```python
from build123d import *

# Parameters (mm, degrees)
F0_W     = 102.87
F0_H     = 13.97
F0_W_2   = 12.3800332606
F0_H_2   = 12.7
F0_W_3   = 3.175
F0_H_3   = 5.08
F0_W_4   = 12.0600665212
F0_W_5   = 0.6399334788
F1_DEPTH = 2.54
F2_DEPTH = 6.35
F3_DEPTH = 3.175
F5_D     = 0.254
F5_DEPTH = 0.636
F6_D     = 0.254


with BuildPart() as f1:
    # F0 (on Top) → F1 (new body)
    with BuildSketch(Plane.XY):
        with Locations((18.0648645937, 6.35)):
            Rectangle(F0_W, F0_H)
        Polygon((-20.3551021457, 0), (-32.7351354063, 0), (-32.7351354063, 12.7), (-20.3551021457, 12.7), (-19.7151686668, 12.7), (-7.6551021457, 12.7), (-7.0151686668, 12.7), (5.0448978543, 12.7), (5.6848313332, 12.7), (17.7448978543, 12.7), (18.3848313332, 12.7), (30.4448978543, 12.7), (31.0848313332, 12.7), (43.1448978543, 12.7), (43.7848313332, 12.7), (55.8448978543, 12.7), (56.4848313332, 12.7), (68.8648645937, 12.7), (68.8648645937, 0), (56.4848313332, 0), (55.8448978543, 0), (43.7848313332, 0), (43.1448978543, 0), (31.0848313332, 0), (30.4448978543, 0), (18.3848313332, 0), (17.7448978543, 0), (5.6848313332, 0), (5.0448978543, 0), (-7.0151686668, 0), (-7.6551021457, 0), (-19.7151686668, 0), align=None, mode=Mode.SUBTRACT)
        with Locations((62.6748479635, 6.35)):
            Rectangle(F0_W_2, F0_H_2)
        with Locations((62.5148645937, 6.35)):
            Rectangle(F0_W_3, F0_H_3, mode=Mode.SUBTRACT)
        with Locations((-26.545118776, 6.35)):
            Rectangle(F0_W_2, F0_H_2)
        with Locations((-26.3851354063, 6.35)):
            Rectangle(F0_W_3, F0_H_3, mode=Mode.SUBTRACT)
        with Locations((-13.6851354063, 6.35)):
            Rectangle(F0_W_4, F0_H_2)
        with Locations((-13.6851354063, 6.35)):
            Rectangle(F0_W_3, F0_H_3, mode=Mode.SUBTRACT)
        with Locations((-0.9851354063, 6.35)):
            Rectangle(F0_W_4, F0_H_2)
        with Locations((-0.9851354063, 6.35)):
            Rectangle(F0_W_3, F0_H_3, mode=Mode.SUBTRACT)
        with Locations((49.8148645937, 6.35)):
            Rectangle(F0_W_4, F0_H_2)
        with Locations((49.8148645937, 6.35)):
            Rectangle(F0_W_3, F0_H_3, mode=Mode.SUBTRACT)
        with Locations((37.1148645937, 6.35)):
            Rectangle(F0_W_4, F0_H_2)
        with Locations((37.1148645937, 6.35)):
            Rectangle(F0_W_3, F0_H_3, mode=Mode.SUBTRACT)
        with Locations((11.7148645937, 6.35)):
            Rectangle(F0_W_4, F0_H_2)
        with Locations((11.7148645937, 6.35)):
            Rectangle(F0_W_3, F0_H_3, mode=Mode.SUBTRACT)
        with Locations((24.4148645937, 6.35)):
            Rectangle(F0_W_4, F0_H_2)
        with Locations((24.4148645937, 6.35)):
            Rectangle(F0_W_3, F0_H_3, mode=Mode.SUBTRACT)
        with Locations((49.8148645937, 6.35)):
            Rectangle(F0_W_3, F0_H_3)
        with Locations((24.4148645937, 6.35)):
            Rectangle(F0_W_3, F0_H_3)
        with Locations((-26.3851354063, 6.35)):
            Rectangle(F0_W_3, F0_H_3)
        with Locations((-0.9851354063, 6.35)):
            Rectangle(F0_W_3, F0_H_3)
        with Locations((-13.6851354063, 6.35)):
            Rectangle(F0_W_3, F0_H_3)
        with Locations((62.5148645937, 6.35)):
            Rectangle(F0_W_3, F0_H_3)
        with Locations((11.7148645937, 6.35)):
            Rectangle(F0_W_3, F0_H_3)
        with Locations((37.1148645937, 6.35)):
            Rectangle(F0_W_3, F0_H_3)
        with Locations((5.3648645937, 6.35)):
            Rectangle(F0_W_5, F0_H_2)
        with Locations((56.1648645937, 6.35)):
            Rectangle(F0_W_5, F0_H_2)
        with Locations((18.0648645937, 6.35)):
            Rectangle(F0_W_5, F0_H_2)
        with Locations((30.7648645937, 6.35)):
            Rectangle(F0_W_5, F0_H_2)
        with Locations((43.4648645937, 6.35)):
            Rectangle(F0_W_5, F0_H_2)
        with Locations((-7.3351354063, 6.35)):
            Rectangle(F0_W_5, F0_H_2)
        with Locations((-20.0351354063, 6.35)):
            Rectangle(F0_W_5, F0_H_2)
    extrude(amount=-F1_DEPTH)

    # F0 (on Top) → F2 (join)
    with BuildSketch(Plane.XY):
        with Locations((18.0648645937, 6.35)):
            Rectangle(F0_W, F0_H)
        Polygon((-20.3551021457, 0), (-32.7351354063, 0), (-32.7351354063, 12.7), (-20.3551021457, 12.7), (-19.7151686668, 12.7), (-7.6551021457, 12.7), (-7.0151686668, 12.7), (5.0448978543, 12.7), (5.6848313332, 12.7), (17.7448978543, 12.7), (18.3848313332, 12.7), (30.4448978543, 12.7), (31.0848313332, 12.7), (43.1448978543, 12.7), (43.7848313332, 12.7), (55.8448978543, 12.7), (56.4848313332, 12.7), (68.8648645937, 12.7), (68.8648645937, 0), (56.4848313332, 0), (55.8448978543, 0), (43.7848313332, 0), (43.1448978543, 0), (31.0848313332, 0), (30.4448978543, 0), (18.3848313332, 0), (17.7448978543, 0), (5.6848313332, 0), (5.0448978543, 0), (-7.0151686668, 0), (-7.6551021457, 0), (-19.7151686668, 0), align=None, mode=Mode.SUBTRACT)
    extrude(amount=F2_DEPTH)

    # F0 (on Top) → F3 (join)
    with BuildSketch(Plane.XY):
        with Locations((-26.3851354063, 6.35)):
            Rectangle(F0_W_3, F0_H_3)
        with Locations((-13.6851354063, 6.35)):
            Rectangle(F0_W_3, F0_H_3)
        with Locations((-0.9851354063, 6.35)):
            Rectangle(F0_W_3, F0_H_3)
        with Locations((11.7148645937, 6.35)):
            Rectangle(F0_W_3, F0_H_3)
        with Locations((24.4148645937, 6.35)):
            Rectangle(F0_W_3, F0_H_3)
        with Locations((37.1148645937, 6.35)):
            Rectangle(F0_W_3, F0_H_3)
        with Locations((49.8148645937, 6.35)):
            Rectangle(F0_W_3, F0_H_3)
        with Locations((62.5148645937, 6.35)):
            Rectangle(F0_W_3, F0_H_3)
        with Locations((56.1648645937, 6.35)):
            Rectangle(F0_W_5, F0_H_2)
        with Locations((43.4648645937, 6.35)):
            Rectangle(F0_W_5, F0_H_2)
        with Locations((30.7648645937, 6.35)):
            Rectangle(F0_W_5, F0_H_2)
        with Locations((18.0648645937, 6.35)):
            Rectangle(F0_W_5, F0_H_2)
        with Locations((5.3648645937, 6.35)):
            Rectangle(F0_W_5, F0_H_2)
        with Locations((-7.3351354063, 6.35)):
            Rectangle(F0_W_5, F0_H_2)
        with Locations((-20.0351354063, 6.35)):
            Rectangle(F0_W_5, F0_H_2)
    extrude(amount=F3_DEPTH)

    # F5 (through all, one way)
    with BuildSketch(Plane(origin=(0, 0, 0), x_dir=(-1, 0, 0), z_dir=(0, 1, 0))):
        with Locations((26.6391354063, 1.5875), (26.1311354063, 1.5875), (13.9391354063, 1.5875), (13.4311354063, 1.5875), (1.2391354063, 1.5875), (0.7311354063, 1.5875), (-11.4608645937, 1.5875), (-11.9688645937, 1.5875), (-24.1608645937, 1.5875), (-24.6688645937, 1.5875), (-36.8608645937, 1.5875), (-37.3688645937, 1.5875), (-49.5608645937, 1.5875), (-50.0688645937, 1.5875), (-62.2608645937, 1.5875), (-62.7688645937, 1.5875)):
            Circle(F5_D / 2)
    extrude(amount=-F5_DEPTH, mode=Mode.SUBTRACT)

    # F6 (through all)
    with Locations(Plane(origin=(0, 0, 0), x_dir=(-1, 0, 0), z_dir=(0, -1, 0))):
        with Locations((-62.7688645937, -1.5875), (-62.2608645937, -1.5875), (-50.0688645937, -1.5875), (-49.5608645937, -1.5875), (-37.3688645937, -1.5875), (-36.8608645937, -1.5875), (-24.6688645937, -1.5875), (-24.1608645937, -1.5875), (-11.9688645937, -1.5875), (-11.4608645937, -1.5875), (0.7311354063, -1.5875), (1.2391354063, -1.5875), (13.4311354063, -1.5875), (13.9391354063, -1.5875), (26.1311354063, -1.5875), (26.6391354063, -1.5875)):
            Hole(F6_D / 2)


solid = f1.part
```
The model under review builds one solid part; all positions refer to its coordinate system, in mm. A direction names the side the tool comes from. Give positions to 0.01 mm unless a question says otherwise; leave off trailing zeros. Write each loop counter-clockwise with the first axis right and the second up, starting at its lowest first coordinate (ties: lowest second). Pieces come first, ordered by that corner, then holes. Notation, with made-up numbers: (48.5, 89) -> (103.5, 89) arc R7 ccw to (103.5, 100) -> close; hole circle Ø3 at (77, 4.25). An arc over 180 degrees is marked (long way). Put each result on its own line as item: value.
(1) To check wall thickness, follow probe 1 along Y at (x, z) = (23, 0.25) (3 decimals); probe 2 along Y at (x, z) = (38.5, 4.75) (3 decimals); probe 3 along X at (y, z) = (10, 5). State the ranges of each line that lie inside material, in increasing order. Write a range as from..to.
Results are:
probe 1: -0.635..0, 3.81..8.89, 12.7..13.335
probe 2: -0.635..0, 12.7..13.335
probe 3: -33.37..-32.74, 68.86..69.5
(2) We need section B-B, the plane x = 53.5. Give the boundary of the cut face in (y, z) (3 decimals), and give its area (3 significant figures).
Results are:
outline: (-0.635, -2.54) -> (13.335, -2.54) -> (13.335, 6.35) -> (12.7, 6.35) -> (12.7, 0) -> (0, 0) -> (0, 6.35) -> (-0.635, 6.35) -> close
area: 43.5 mm²
(3) We need section C-C, the plane y = 7.25. State how many separate pieces and enclosed holes the cut face has, and give its area (3 significant figures).
Results are:
separate pieces: 1
enclosed holes: 16
area: 363 mm²
(4) We need section A-A, the plane z = 5.25. Give the boundary of the cut face in (x, y) (3 decimals).
Results are:
outline: (-33.37, -0.635) -> (69.5, -0.635) -> (69.5, 13.335) -> (-33.37, 13.335) -> close; hole (-32.735, 0) -> (68.865, 0) -> (68.865, 12.7) -> (-32.735, 12.7) -> close
(5) The part is to be moulded in two halves that separate along X. For faces 1 (the flat face through (17, -0.635, 2)), 2 (the flat face through (48.227, 6, 2)), say which applies: pulls with the +X half, pulls with the -X half, needs draft (parallel to the pull), parting line crosses it, or undercut.
Results are:
face 1: needs draft
face 2: undercut
(6) For pin 1 Ø1 at (x, y) = (-27, 6) entering from +Z (3 decimals), flat-tipped, find the tip position at first contact; note if it passes through.
Results are:
pin 1: z = 3.175
(7) Tool access review of faces 3 (the flat face through (43.785, 6, 2)), 4 (the flat face through (17, 13.335, 2)): name each direction out of +Z, -Z, +X, -X, +Y, -Y from which nothing blocks a thin tool from reaching the whole face with its end or side.
Results are:
face 3: +Z
face 4: +Z, -Z, +X, -X, +Y
